For this review, take the finished solid that the model builds, in its own axes (mm). A direction names the side the tool comes from. Give positions to 0.01 mm unless a question says otherwise; leave off trailing zeros. Loops run counter-clockwise (first coordinate to the right, second up) from the corner with the lowest first, then second, coordinate; pieces in that order, holes last.
```python
from build123d import *

# Parameters (mm, degrees)
F0_R     = 3.96875
F1_DEPTH = 19.05
F3_DEPTH = 127


with BuildPart() as f1:
    # F0 (on Front) → F1 (new body)
    with BuildSketch(Plane.XZ):
        with BuildLine():
            ThreePointArc((0, -9.525), (6.7351920908, -6.7351920908), (9.525, 0))
            ThreePointArc((9.525, 0), (6.7351920908, 6.7351920908), (0, 9.525))
            ThreePointArc((0, 9.525), (-6.7351920908, 6.7351920908), (-9.525, 0))
            ThreePointArc((-9.525, 0), (-6.7351920908, -6.7351920908), (0, -9.525))
        make_face()
        Circle(F0_R, mode=Mode.SUBTRACT)
        with BuildLine():
            Line((9.525, -9.525), (9.525, 0))
            ThreePointArc((9.525, 0), (6.7351920908, -6.7351920908), (0, -9.525))
            Line((0, -9.525), (9.525, -9.525))
        make_face()
        with BuildLine():
            ThreePointArc((0, 9.525), (6.7351920908, 6.7351920908), (9.525, 0))
            Line((9.525, 0), (9.525, 9.525))
            Line((9.525, 9.525), (0, 9.525))
        make_face()
        with BuildLine():
            ThreePointArc((-9.525, 0), (-6.7351920908, 6.7351920908), (0, 9.525))
            Line((0, 9.525), (-9.525, 9.525))
            Line((-9.525, 9.525), (-9.525, 0))
        make_face()
        with BuildLine():
            Line((-9.525, -9.525), (0, -9.525))
            ThreePointArc((0, -9.525), (-6.7351920908, -6.7351920908), (-9.525, 0))
            Line((-9.525, 0), (-9.525, -9.525))
        make_face()
    extrude(amount=F1_DEPTH)

    # F2 (on face) → F3 (cut)
    with BuildSketch(Plane.YZ.offset(9.525)):
        Polygon((-14.3871692356, 13.1968459708), (-9.525, 8.3346767351), (-4.6628307644, 13.1968459708), align=None)
    extrude(amount=-F3_DEPTH, mode=Mode.SUBTRACT)

    # F4 (on Right) → F5 (revolve, cut)
    with BuildSketch(Plane.YZ):
        Polygon((-19.05, 15.1654964413), (-19.05, 9.525), (-17.5386335336, 15.1654964413), align=None)
    revolve(axis=Axis((0, -19.05, 0), (0, -1, 0)), mode=Mode.SUBTRACT)

    # F6 (on Right) → F7 (revolve, cut)
    with BuildSketch(Plane.YZ):
        Polygon((-1.3839481467, 14.6899647984), (0, 9.525), (0, 14.6899647984), align=None)
    revolve(axis=Axis((0, 0, 0), (0, -1, 0)), mode=Mode.SUBTRACT)


solid = f1.part
```
Q1. Consider section A-A on y = -13.5. Give the boundary of the cut face in (x, z) (1 decimal).
Answers:
outline: (-9.5, -9.5) - (9.5, -9.5) - (9.5, 9.5) - (-9.5, 9.5) - close; hole circle Ø7.9 at (0, 0)
Q2. Machinability: for faces 4 (the flat face through (0.13, -10.13, 8.94)), 5 (the flat face through (0, -4, 9.525)), which of the approach directions +Z, -Z, +X, -X, +Y, -Y give a long, thin tool a straight path to every point of the face, cutting with its end or side? Answer none if there is none.
Answers:
face 4: +Z, +X, -X
face 5: +Z, +X, -X, +Y, -Y
Q3. For probe 1 along Z at (x, y) = (0, -5) (3 decimals); probe 2 along Z at (x, y) = (-3, -7.75) (3 decimals); probe 3 along X at (y, z) = (-3, -2.25) (3 decimals), list the stretches that pass through material, from the lowest coordinate up.
Answers:
probe 1: z = -9.525 to -3.969, 3.969 to 9.525
probe 2: z = -9.525 to -2.598, 2.598 to 9.525
probe 3: x = -9.525 to -3.269, 3.269 to 9.525
Q4. Mouldability with a two-part tool opening along Z and no side actions: class faces 1 (the flat face through (4, 0, -2)), 2 (the cylindrical face through (-0.86, -9.392, -3.874)), 3 (the flat face through (0.13, -8.94, 8.92)) as +Z half, -Z half, draft (parallel to the pull), parting line (faces both ways), or undercut.
Answers:
face 1: draft
face 2: undercut
face 3: +Z half
